from build123d import *

# Parameters (mm, degrees)
SKETCH_1_W          = 50
SKETCH_1_H          = 20
EXTRUDE_1_DEPTH     = 3
SKETCH_2_W          = 50
SKETCH_2_H          = 12
EXTRUDE_2_DEPTH     = 6
SKETCH_5_W          = 50
SKETCH_5_H          = 9
CUT_EXTRUDE_2_DEPTH = 3
EXTRUDE_3_DEPTH     = 3
EXTRUDE_4_DEPTH     = 55
SKETCH_12_W         = 32.35533906
SKETCH_12_H         = 3
EXTRUDE_6_DEPTH     = 10
EXTRUDE_7_DEPTH     = 3
EXTRUDE_8_DEPTH     = 3
SKETCH_15_R         = 1.65
CUT_EXTRUDE_3_DEPTH = 3


with BuildPart() as part:
    # 草图1 → 凸台-拉伸1 (new body)
    with BuildSketch(Plane.XY):
        Rectangle(SKETCH_1_W, SKETCH_1_H)
        with BuildLine():
            Line((-3.85, 2.5), (3.85, 2.5))
            ThreePointArc((3.85, 2.5), (4.404700196, 2.667949706), (4.773076923, 3.115384615))
            ThreePointArc((4.773076923, 3.115384615), (20.35, 0), (4.773076923, -3.115384615))
            ThreePointArc((4.773076923, -3.115384615), (4.404700196, -2.667949706), (3.85, -2.5))
            Line((3.85, -2.5), (-3.85, -2.5))
            ThreePointArc((-3.85, -2.5), (-4.404700196, -2.667949706), (-4.773076923, -3.115384615))
            ThreePointArc((-4.773076923, -3.115384615), (-20.35, 0), (-4.773076923, 3.115384615))
            ThreePointArc((-4.773076923, 3.115384615), (-4.404700196, 2.667949706), (-3.85, 2.5))
        make_face(mode=Mode.SUBTRACT)
        with BuildLine():
            Line((3.25, 5.5), (-3.25, 5.5))
            ThreePointArc((-3.25, 5.5), (-5, 7.25), (-3.25, 9))
            Line((-3.25, 9), (3.25, 9))
            ThreePointArc((3.25, 9), (5, 7.25), (3.25, 5.5))
        make_face(mode=Mode.SUBTRACT)
    extrude(amount=EXTRUDE_1_DEPTH)

    # 草图2 → 凸台-拉伸2 (add)
    with BuildSketch(Plane(origin=(0, 10, 0), x_dir=(1, 0, 0), z_dir=(0, 1, 0))):
        with Locations((0, -6)):
            Rectangle(SKETCH_2_W, SKETCH_2_H)
    extrude(amount=EXTRUDE_2_DEPTH)

    # 草图5 → 切除-拉伸2 (cut)
    with BuildSketch(Plane.XZ.offset(-10)):
        with Locations((0, 7.5)):
            Rectangle(SKETCH_5_W, SKETCH_5_H)
    extrude(amount=-CUT_EXTRUDE_2_DEPTH, mode=Mode.SUBTRACT)

    # 草图9 → 凸台-拉伸3 (add)
    with BuildSketch(Plane(origin=(0, 16, 0), x_dir=(1, 0, 0), z_dir=(0, 1, 0))):
        Polygon((25, 0), (0, 25), (-25, 0), align=None)
    extrude(amount=-EXTRUDE_3_DEPTH)

    # 草图11 → 凸台-拉伸4 (add)
    with BuildSketch(Plane(origin=(0, 16, 0), x_dir=(1, 0, 0), z_dir=(0, 1, 0))):
        Polygon((0, 25), (2.121320344, 22.878679656), (-22.878679656, -2.121320344), (-25, 0), align=None)
    extrude(amount=EXTRUDE_4_DEPTH)

    # 草图12 → 凸台-拉伸6 (add)
    with BuildSketch(Plane(origin=(-10.378679656, 0, -10.378679656), x_dir=(0.707106781, 0, -0.707106781), z_dir=(0.707106781, 0, 0.707106781))):
        with Locations((-1.5, 69.5)):
            Rectangle(SKETCH_12_W, SKETCH_12_H)
    extrude(amount=EXTRUDE_6_DEPTH)

    # 草图13 → 凸台-拉伸7 (add)
    with BuildSketch(Plane(origin=(12.5, 0, -12.5), x_dir=(-0.707106781, 0, -0.707106781), z_dir=(0.707106781, 0, -0.707106781))):
        Polygon((14.67766953, 16), (14.67766953, 46), (-0.32233047, 16), align=None)
        Polygon((14.67766953, 46), (14.67766953, 71), (4.67766953, 71), (4.67766953, 68), align=None)
    extrude(amount=-EXTRUDE_7_DEPTH)

    # 草图14 → 凸台-拉伸8 (add)
    with BuildSketch(Plane(origin=(-12.5, 0, 12.5), x_dir=(0.707106781, 0, 0.707106781), z_dir=(-0.707106781, 0, 0.707106781))):
        Polygon((-14.67766953, 46), (-14.67766953, 16), (-4.67766953, 16), align=None)
        Polygon((-14.67766953, 68), (-14.67766953, 46), (-4.67766953, 68), align=None)
    extrude(amount=-EXTRUDE_8_DEPTH)

    # 草图15 → 切除-拉伸3 (cut)
    with BuildSketch(Plane.XZ.offset(-68)):
        with Locations((0.227922061, -13.914213562)):
            Circle(SKETCH_15_R)
        with Locations((-13.914213562, 0.227922061)):
            Circle(SKETCH_15_R)
    extrude(amount=-CUT_EXTRUDE_3_DEPTH, mode=Mode.SUBTRACT)


solid = part.part
Part model, mm, in its own coordinate system. A direction names the side the tool comes from. Give positions to 0.01 mm unless a question says otherwise; leave off trailing zeros. Loops run counter-clockwise (first coordinate to the right, second up) from the corner with the lowest first, then second, coordinate; pieces in that order, holes last.
(1) Pin check, flat tips, straight feed: pin 1 (10 mm diameter, centred on x = -14.5, y = 49.5, fed in from -Z); pin 2 (11.5 mm diameter, centred on x = -8.5, y = 2, fed in from +Z); pin 3 (3 mm diameter, centred on x = -13.91, z = 0.23, fed in from +Y); pin 4 (8 mm diameter, centred on x = -18.5, z = -10, fed in from +Y). Stop position of each tip, or through.
Return value:
pin 1: stops at z = -15.5
pin 2: stops at z = 3
pin 3: stops at y = 16
pin 4: stops at y = 71
(2) Band-saw the part on B-B (z = 5). Write the cut outline in (x, y).
Return value:
outline: (-25, 13) - (25, 13) - (25, 16) - (-15.76, 16) - (-15.76, 24.79) - (-20, 33.79) - (-20, 16) - (-25, 16) - close; (-20, 54.96) - (-15.76, 61.56) - (-15.76, 68) - (-11.62, 68) - (-11.62, 71) - (-20, 71) - close
(3) Band-saw the part on C-C (y = 58). Write the cut outline in (x, z), and give its area (3 significant figures).
Return value:
outline: (-25, 0) - (0, -25) - (5.98, -19.02) - (3.86, -16.9) - (0, -20.76) - (-20.76, 0) - (-16.9, 3.86) - (-19.02, 5.98) - close
area: 139 mm2
(4) Band-saw the part on A-A (y = 0). Write the cut outline in (x, z).
Return value:
outline: (-25, 0) - (-20.35, 0) - (-20.35, 3) - (-25, 3) - close; (20.35, 0) - (25, 0) - (25, 3) - (20.35, 3) - close
(5) Drill centre lines: line 1 along Y through (x, z) = (-12.25, 1.4); line 2 along Y through (x, z) = (-6, -6); line 3 along Y through (x, z) = (16.5, 1). Where is each one in solid material? Low to high.
Return value:
line 1: y = -10 to -8.1, 8.1 to 16, 68 to 71
line 2: y = 13 to 16, 68 to 71
line 3: y = -10 to -6.9, 6.9 to 16
(6) Band-saw the part on D-D (z = -3.5). Write the cut outline in (x, y).
Return value:
outline: (-21.5, 13) - (21.5, 13) - (21.5, 16) - (-17.26, 16) - (-17.26, 68) - (-3.12, 68) - (-3.12, 71) - (-21.5, 71) - close
(7) Pull direction X, two halves, no side cores. Call faces 6 (the flat face through (-18.25, 30.79, 4.66)), 7 (the flat face through (0, 2.5, 1)), 8 (the flat face through (0, 4, 0)): pulls with the +X half, pulls with the -X half, needs draft (parallel to the pull), parting line crosses it, or undercut.
Return value:
face 6: pulls with the +X half
face 7: undercut
face 8: needs draft
(8) 3-axis set-ups, long thin cutter, end or side, ignore diameter. For faces 1 (the flat face through (2.014, 62.043, -18.744)), 2 (the flat face through (-18.843, 24.543, 1.915)), 3 (the flat face through (6.3, 31.21, -16.6)), 4 (the flat face through (0, 13, 8)), 5 (the flat face through (-10.233, 41.636, -10.524)): which of +Z, -Z, +X, -X, +Y, -Y reach the whole face in a straight line?
Return value:
face 1: +Z
face 2: +X
face 3: +Z, +X
face 4: +Z, +X, -X, -Y
face 5: none
